For this review, take the finished solid that the model builds, in its own axes (mm). Coordinates: 2 decimals unless noted, no trailing zeros. Order: outer loops, then holes, each group sorted by start corner. A loop starts at its lowest first (then second) coordinate and runs counter-clockwise, first axis right, second up. Notation, with made-up numbers: (26.5, -21.75) -> (32.5, -21.75) arc R12 ccw to (32.5, -16.75) -> close; hole circle Ø2 at (-36, 30.25). An arc over 180 degrees is marked (long way). Write item = value, one per line. Start each with the question number.
1) Consider section A-A on z = 1.3. State how many separate pieces and enclosed holes the cut face has, and give its area (3 significant figures).
2) Consider section C-C on y = -48.5. Give the boundary of the cut face in (x, z).
3) Consider section D-D on y = -2. Give the boundary of the cut face in (x, z), and give its area (3 significant figures).
4) Consider section B-B on x = 23. Give the boundary of the cut face in (y, z).
5) Wall thickness on probe 1 along Y at (x, z) = (32.95, 0.95); probe 2 along Y at (x, z) = (-22.7, 0.95); probe 3 along Y at (x, z) = (32.5, 0.25): over which ranges is each line inside the solid? List them lowest first. Write a range as [from, to].
6) Draft analysis for pull direction X (two halves, no side actions). For faces 1 (the face through (22.87, 3.24, 0.25)), 2 (the face through (32, 7, 0.07)), 3 (the face through (22, 0, 0.5)), state which applies: +X half, -X half, draft (parallel to the pull), parting line (faces both ways), or undercut.
7) Insertion check: pin 1 Ø0.8 at (x, z) = (-32, 1) entering from +Y; pin 2 Ø3 at (x, y) = (-33, 7.5) entering from -Z (3 decimals); pin 3 Ø0.8 at (y, z) = (1, 1) entering from -X. Each pin has a flat end and moves straight along its axis. Give the tip position at first contact, or say it passes through.
from build123d import *

# Parameters (mm, degrees)
SKETCH1_W               = 120
SKETCH1_H               = 60.9
BOSS_EXTRUDE1_DEPTH     = 1.61
CUT_EXTRUDE1_DEPTH      = 0.5
SKETCH3_W               = 4
SKETCH3_H               = 1.54
BOSS_EXTRUDE2_DEPTH     = 4
SKETCH5_W               = 4
SKETCH5_H               = 1.47
BOSS_EXTRUDE3_DEPTH     = 4
SKETCH7_R               = 0.75
CUT_EXTRUDE3_DEPTH      = 1.07
CUT_EXTRUDE3_DEPTH_BACK = 2.54
FILLET1_R               = 1.2
FILLET2_R               = 1.2
SKETCH8_R               = 0.7
CUT_EXTRUDE4_DEPTH      = 2.61
SKETCH13_W              = 60.9
SKETCH13_H              = 120
CUT_EXTRUDE5_DEPTH      = 0.04
SKETCH14_R              = 0.75
BOSS_EXTRUDE4_DEPTH     = 0.03
SKETCH15_R              = 0.75
CUT_EXTRUDE6_DEPTH      = 0.005


with BuildPart() as part:
    # Sketch1 → Boss-Extrude1 (new body)
    with BuildSketch(Plane(origin=(0, 0, 0), x_dir=(0, 1, 0), z_dir=(0, 0, 1))):
        Rectangle(SKETCH1_W, SKETCH1_H)
    extrude(amount=BOSS_EXTRUDE1_DEPTH)

    # Sketch2 → Cut-Extrude1 (cut)
    with BuildSketch(Plane(origin=(0, 0, 0), x_dir=(1, 0, 0), z_dir=(0, 0, -1))):
        Polygon((28.481704711, 0), (17.415141609, 6.389283186), (17.415141609, -6.389283186), align=None)
    extrude(amount=-CUT_EXTRUDE1_DEPTH, mode=Mode.SUBTRACT)

    # Sketch3 → Boss-Extrude2 (add)
    with BuildSketch(Plane(origin=(-30.45, 0, 0), x_dir=(0, -1, 0), z_dir=(-1, 0, 0))):
        with Locations((-7, 0.805)):
            Rectangle(SKETCH3_W, SKETCH3_H)
        with Locations((7, 0.805)):
            Rectangle(SKETCH3_W, SKETCH3_H)
    extrude(amount=BOSS_EXTRUDE2_DEPTH)

    # Sketch5 → Boss-Extrude3 (add)
    with BuildSketch(Plane.YZ.offset(30.45)):
        with Locations((7, 0.805)):
            Rectangle(SKETCH5_W, SKETCH5_H)
        with Locations((-7, 0.805)):
            Rectangle(SKETCH5_W, SKETCH5_H)
    extrude(amount=BOSS_EXTRUDE3_DEPTH)

    # Sketch7 → Cut-Extrude3 (cut, two sides)
    with BuildSketch(Plane.XY.offset(1.54)) as cut_extrude3_sk:
        with Locations((32.95, 7)):
            Circle(SKETCH7_R)
        with Locations((32.95, -7)):
            Circle(SKETCH7_R)
        with Locations((-32.95, -7)):
            Circle(SKETCH7_R)
        with Locations((-32.95, 7)):
            Circle(SKETCH7_R)
    extrude(amount=CUT_EXTRUDE3_DEPTH, mode=Mode.SUBTRACT)
    extrude(cut_extrude3_sk.sketch, amount=-CUT_EXTRUDE3_DEPTH_BACK, mode=Mode.SUBTRACT)

    # Fillet1
    fillet1_edges = [part.edges().sort_by_distance(p)[0] for p in [
        (-30.45, 5, 0.805),
        (-30.45, 9, 0.805),
        (-30.45, -9, 0.805),
        (-30.45, -5, 0.805),
        (30.45, 9, 0.805),
        (30.45, 5, 0.805),
        (30.45, -5, 0.805),
        (30.45, -9, 0.805),
    ]]
    fillet(fillet1_edges, radius=FILLET1_R)

    # Fillet2
    fillet2_edges = [part.edges().sort_by_distance(p)[0] for p in [
        (-34.45, 9, 0.805),
        (-34.45, 5, 0.805),
        (-34.45, -5, 0.805),
        (-34.45, -9, 0.805),
        (34.45, 5, 0.805),
        (34.45, 9, 0.805),
        (34.45, -9, 0.805),
        (34.45, -5, 0.805),
    ]]
    fillet(fillet2_edges, radius=FILLET2_R)

    # Sketch8 → Cut-Extrude4 (cut, through all)
    with BuildSketch(Plane(origin=(0, 0, 0), x_dir=(1, 0, 0), z_dir=(0, 0, -1))):
        with Locations((-22.7, 0)):
            Circle(SKETCH8_R)
    extrude(amount=-CUT_EXTRUDE4_DEPTH, mode=Mode.SUBTRACT)

    # Sketch13 → Cut-Extrude5 (cut)
    with BuildSketch(Plane.XY.offset(1.61)):
        Rectangle(SKETCH13_W, SKETCH13_H)
    extrude(amount=-CUT_EXTRUDE5_DEPTH, mode=Mode.SUBTRACT)

    # Sketch14 → Boss-Extrude4 (add)
    with BuildSketch(Plane.XY.offset(1.54)):
        with BuildLine():
            Line((31.65, -9), (33.25, -9))
            ThreePointArc((33.25, -9), (34.098528137, -8.648528137), (34.45, -7.8))
            Line((34.45, -7.8), (34.45, -6.2))
            ThreePointArc((34.45, -6.2), (34.098528137, -5.351471863), (33.25, -5))
            Line((33.25, -5), (31.65, -5))
            ThreePointArc((31.65, -5), (30.801471863, -4.648528137), (30.45, -3.8))
            Line((30.45, -3.8), (30.45, -10.2))
            ThreePointArc((30.45, -10.2), (30.801471863, -9.351471863), (31.65, -9))
        make_face()
        with Locations((32.95, -7)):
            Circle(SKETCH14_R, mode=Mode.SUBTRACT)
        with BuildLine():
            Line((34.45, 6.2), (34.45, 7.8))
            ThreePointArc((34.45, 7.8), (34.098528137, 8.648528137), (33.25, 9))
            Line((33.25, 9), (31.65, 9))
            ThreePointArc((31.65, 9), (30.801471863, 9.351471863), (30.45, 10.2))
            Line((30.45, 10.2), (30.45, 3.8))
            ThreePointArc((30.45, 3.8), (30.801471863, 4.648528137), (31.65, 5))
            Line((31.65, 5), (33.25, 5))
            ThreePointArc((33.25, 5), (34.098528137, 5.351471863), (34.45, 6.2))
        make_face()
        with Locations((32.95, 7)):
            Circle(SKETCH14_R, mode=Mode.SUBTRACT)
    extrude(amount=BOSS_EXTRUDE4_DEPTH)

    # Sketch15 → Cut-Extrude6 (cut)
    with BuildSketch(Plane.XY.offset(1.575)):
        with BuildLine():
            Line((-34.45, 7.8), (-34.45, 6.2))
            ThreePointArc((-34.45, 6.2), (-34.098528137, 5.351471863), (-33.25, 5))
            Line((-33.25, 5), (-31.65, 5))
            ThreePointArc((-31.65, 5), (-30.801471863, 4.648528137), (-30.45, 3.8))
            Line((-30.45, 3.8), (-30.45, 10.2))
            ThreePointArc((-30.45, 10.2), (-30.801471863, 9.351471863), (-31.65, 9))
            Line((-31.65, 9), (-33.25, 9))
            ThreePointArc((-33.25, 9), (-34.098528137, 8.648528137), (-34.45, 7.8))
        make_face()
        with Locations((-32.95, 7)):
            Circle(SKETCH15_R, mode=Mode.SUBTRACT)
        with BuildLine():
            Line((-34.45, -6.2), (-34.45, -7.8))
            ThreePointArc((-34.45, -7.8), (-34.098528137, -8.648528137), (-33.25, -9))
            Line((-33.25, -9), (-31.65, -9))
            ThreePointArc((-31.65, -9), (-30.801471863, -9.351471863), (-30.45, -10.2))
            Line((-30.45, -10.2), (-30.45, -3.8))
            ThreePointArc((-30.45, -3.8), (-30.801471863, -4.648528137), (-31.65, -5))
            Line((-31.65, -5), (-33.25, -5))
            ThreePointArc((-33.25, -5), (-34.098528137, -5.351471863), (-34.45, -6.2))
        make_face()
        with Locations((-32.95, -7)):
            Circle(SKETCH15_R, mode=Mode.SUBTRACT)
    extrude(amount=-CUT_EXTRUDE6_DEPTH, mode=Mode.SUBTRACT)


solid = part.part
Answer sheet:
q1.separate_pieces = 1
q1.enclosed_holes = 5
q1.area = 7,360 mm2
q2.outline = (-30.45, 0) -> (30.45, 0) -> (30.45, 1.57) -> (-30.45, 1.57) -> close
q3.outline = (-30.45, 0) -> (17.42, 0) -> (17.42, 0.5) -> (25.02, 0.5) -> (25.02, 0) -> (30.45, 0) -> (30.45, 1.57) -> (-30.45, 1.57) -> close
q3.area = 91.8 mm2
q4.outline = (-60, 0) -> (-3.16, 0) -> (-3.16, 0.5) -> (3.16, 0.5) -> (3.16, 0) -> (60, 0) -> (60, 1.57) -> (-60, 1.57) -> close
q5.probe_1 = [-9, -7.75], [-6.25, -5], [5, 6.25], [7.75, 9]
q5.probe_2 = [-60, -0.7], [0.7, 60]
q5.probe_3 = [-9, -7.6], [-6.4, -5], [5, 6.4], [7.6, 9]
q6.face_1 = undercut
q6.face_2 = draft
q6.face_3 = undercut
q7.pin_1 = 9
q7.pin_2 = 0.035
q7.pin_3 = -30.45
